Design review of the part built by this model. Coordinates are the model's own, in mm. A direction names the side the tool comes from. Coordinates: 2 decimals unless noted, no trailing zeros. Loops run counter-clockwise (first coordinate to the right, second up) from the corner with the lowest first, then second, coordinate; pieces in that order, holes last. Notation, with made-up numbers: (-12.5, 14) - (42.5, 14) arc R18 ccw to (42.5, 37) - close; hole circle Ø6 at (87, -21). An arc over 180 degrees is marked (long way). One line per question, with ' | ' between items.
Autodesk Inventor part; units mm, degrees
ref_plane "YZ Plane" through (0, 0, 0) normal (1, 0, 0) x (0, 1, 0)
ref_plane "XZ Plane" through (0, 0, 0) normal (0, 1, 0) x (-1, 0, 0)
ref_plane "XY Plane" through (0, 0, 0) normal (0, 0, 1) x (1, 0, 0)
sketch "Sketch1" plane through (0, 0, 0) normal (0, 0, 1) x (1, 0, 0)
  circle A0 centre (0, 0) radius 9.5
  arc A1 (-3.096, -4.5458) -> (5.2116, 1.7576) centre (0, 0) ccw
  point P0 (0, 0)
  dimension "d0" = 19
extrude "Extrusion1" add sketch "Sketch1" along normal blind 10.5
sketch "Sketch2" plane through (0, 0, 10.5) normal (0, 0, 1) x (1, 0, 0)
  circle A0 centre (0, 0) radius 9.5
  line L0 (9.5, 0) -> (7, 0)
  circle A1 centre (7, 0) radius 2.125
  point P0 (0, 0)
  dimension "d3" = 2.5
  dimension "d4" = 4.25
extrude "Extrusion2" cut sketch "Sketch2" against normal blind 5 contours A1
sketch "Sketch3" plane through (0, 0, 0) normal (0, 0, -1) x (-1, 0, 0)
  circle A0 centre (0, 0) radius 5
  circle A1 centre (0, 0) radius 9.5
  circle A2 centre (0, 0) radius 8.5
  point P0 (0, 0)
  dimension "d7" = 17
extrude "Extrusion3" add sketch "Sketch3" along normal blind 3 contours A0 | A2
sketch "Sketch5" plane through (0, 0, -3) normal (0, 0, -1) x (-1, 0, 0)
  circle A0 centre (0, 0) radius 1
  dimension "d13" = 2
extrude "Extrusion5" cut sketch "Sketch5" against normal blind 10
properties part number "RotationDisk"
Q1. Take a section at B-B (x = 0). Give the boundary of the cut face in (y, z), plus the area to 4 significant figures.
Returned:
outline: (-9.5, 0) - (-8.5, 0) - (-8.5, -3) - (-1, -3) - (-1, 7) - (1, 7) - (1, -3) - (8.5, -3) - (8.5, 0) - (9.5, 0) - (9.5, 10.5) - (-9.5, 10.5) - close | area: 230.5 mm²
Q2. For pin 1 (6 mm diameter, centred on x = -7, z = 3, fed in from -Y); pin 2 (2 mm diameter, centred on x = -3.5, z = 9, fed in from +Y); pin 3 (1.5 mm diameter, centred on y = 2, z = 8, fed in from -X), all flat-tipped, find the tip position at first contact; note any pin that passes through.
Returned:
pin 1: stops at y = -8.62 | pin 2: stops at y = 9.17 | pin 3: stops at x = -9.42
Q3. Take a section at C-C (z = 5.75). Give the boundary of the cut face in (x, y) (3 decimals).
Returned:
outline: circle Ø19 at (0, 0); hole circle Ø2 at (0, 0); hole circle Ø4.25 at (7, 0)
Q4. Tool access review of faces 1 (the cylindrical face through (8.963, -0.814, 8.035)), 2 (the flat face through (-2, 0, -3)), 3 (the cylindrical face through (0, -1, 2)): name each direction out of +Z, -Z, +X, -X, +Y, -Y from which nothing blocks a thin tool from reaching the whole face with its end or side.
Returned:
face 1: +Z | face 2: -Z, +X, -X, +Y, -Y | face 3: -Z
Q5. Draft analysis for pull direction X (two halves, no side actions). For faces 4 (the cylindrical face through (-4.57, -7.167, -1.479)), 5 (the flat face through (0, 0, 10.5)), 6 (the flat face through (7, 0, 5.5)), state which applies: +X half, -X half, draft (parallel to the pull), parting line (faces both ways), or undercut.
Returned:
face 4: parting line | face 5: draft | face 6: undercut
Q6. To check wall thickness, follow line 1 along Y through (x, z) = (0, 1.5); line 2 along Z through (x, y) = (7.25, -4.5); line 3 along Y through (x, z) = (7, 8.1) (3 decimals). State the ranges of each line that lie inside material, in increasing order.
Returned:
line 1: y = -9.5 to -1, 1 to 9.5 | line 2: z = 0 to 10.5 | line 3: y = -6.423 to -2.125, 2.125 to 6.423
Q7. Take a section at D-D (z = -1.5). Give the boundary of the cut face in (x, y).
Returned:
outline: circle Ø17 at (0, 0); hole circle Ø2 at (0, 0)
Q8. Take a section at A-A (y = 0). Give the boundary of the cut face in (x, z) (3 decimals).
Returned:
outline: (-9.5, 0) - (-8.5, 0) - (-8.5, -3) - (-1, -3) - (-1, 7) - (1, 7) - (1, -3) - (8.5, -3) - (8.5, 0) - (9.5, 0) - (9.5, 10.5) - (9.125, 10.5) - (9.125, 5.5) - (4.875, 5.5) - (4.875, 10.5) - (-9.5, 10.5) - close
